The model under review builds one solid part; all positions refer to its coordinate system, in mm. A direction names the side the tool comes from. Give positions to 0.01 mm unless a question says otherwise; leave off trailing zeros. Write each loop counter-clockwise with the first axis right and the second up, starting at its lowest first coordinate (ties: lowest second). Pieces come first, ordered by that corner, then holes. Notation, with made-up numbers: (17.5, 11) - (44.5, 11) arc R24 ccw to (44.5, 41) - close; hole circle Ø9 at (82, -36). An arc over 180 degrees is marked (long way). Write item = value, one per line.
```python
from build123d import *

# Parameters (mm, degrees)
BOSS_EXTRUDE1_DEPTH = 1.8
FILLET1_R           = 0.5
SKETCH2_R           = 1.75
BOSS_EXTRUDE3_DEPTH = 1.8
FILLET2_R           = 3


with BuildPart() as part:
    # Sketch1 → Boss-Extrude1 (new body)
    with BuildSketch(Plane.XY):
        with BuildLine():
            Line((0, 4.5), (0, 6.5))
            Line((0, 6.5), (6, 6.5))
            Line((6, 6.5), (6, 10.5))
            Line((6, 10.5), (10, 14.5))
            Line((10, 14.5), (10, 83.5))
            Line((10, 83.5), (16.4, 83.5))
            ThreePointArc((16.4, 83.5), (17.2719581, 81.425344658), (17.601960582, 79.199226044))
            Line((17.601960582, 79.199226044), (18.25, 49.5))
            Line((18.25, 49.5), (12, 49.5))
            Line((12, 49.5), (12, 37))
            add(Edge.make_bspline(
                [(12, 37), (12, 35.742192932), (12.5, 34.153450807), (12.5, 32.15)],
                knots=[0, 0, 0, 0, 1, 1, 1, 1], degree=3))
            Line((12.5, 32.15), (12.5, 2.89))
            ThreePointArc((12.5, 2.89), (11.653538598, 0.846461402), (9.61, 0))
            ThreePointArc((9.61, 0), (4.304293167, 1.180712741), (0, 4.5))
        make_face()
    extrude(amount=BOSS_EXTRUDE1_DEPTH)

    # Fillet1
    fillet1_edges = [part.edges().sort_by_distance(p)[0] for p in [
        (0, 4.5, 0.9),
        (0, 6.5, 0.9),
        (6, 6.5, 0.9),
        (6, 10.5, 0.9),
        (10, 14.5, 0.9),
        (10, 83.5, 0.9),
        (18.25, 49.5, 0.9),
        (12, 49.5, 0.9),
    ]]
    fillet(fillet1_edges, radius=FILLET1_R)

    # Sketch2 → Boss-Extrude3 (add)
    with BuildSketch(Plane.XY):
        with BuildLine():
            Line((7, -2.499596966), (7, 0.500403034))
            Line((7, 0.500403034), (11, 0.500403034))
            Line((11, 0.500403034), (11.824045318, -1.578286292))
            ThreePointArc((11.824045318, -1.578286292), (9.968981185, -4.955214332), (7, -2.499596966))
        make_face()
        with Locations((9.5, -2.499596966)):
            Circle(SKETCH2_R, mode=Mode.SUBTRACT)
    extrude(amount=BOSS_EXTRUDE3_DEPTH)

    # Fillet2
    fillet2_edges = [part.edges().sort_by_distance(p)[0] for p in [
        (16.4, 83.5, 0.9),
    ]]
    fillet(fillet2_edges, radius=FILLET2_R)


solid = part.part
```
1. Insertion check: P1, Ø0.9, axis at x = 16.5, z = 1, coming from the -Y side; P2, Ø0.5, axis at y = 9, z = 1, coming from the -X side; P3, Ø0.5, axis at y = -1.5, z = 1, coming from the -X side. Each pin has a flat end and moves straight along its axis. Give the tip position at first contact, or say it passes through.
Findings below:
P1 = 49.5
P2 = 6
P3 = 7
2. Take a section at A-A on y = 38. Give the boundary of the cut face in (x, z), and give its area (3 significant figures).
Findings below:
outline = (10, 0) - (12, 0) - (12, 1.8) - (10, 1.8) - close
area = 3.60 mm²
3. For line 1 (Y direction, x = 9.25, z = 0.95); line 2 (X direction, y = 32.5, z = 0.6) (3 decimals); line 3 (Y direction, x = 9.5, z = 1.35), list the stretches that pass through material, from the lowest coordinate up. Write a range as from..to.
Findings below:
line_1 = -4.99..-4.23, -0.77..13.75
line_2 = 10..12.495
line_3 = -5..-4.25, -0.75..14
4. Take a section at B-B on x = 3. Give the boundary of the cut face in (y, z).
Findings below:
outline = (1.89, 0) - (6.5, 0) - (6.5, 1.8) - (1.89, 1.8) - close
5. Draft analysis for pull direction Y (two halves, no side actions). For faces 1 (the flat face through (11.43, -0.58, 0.89)), 2 (the flat face through (8, 12.5, 0.9)), 3 (the flat face through (7, -1, 1)), state which applies: +Y half, -Y half, draft (parallel to the pull), parting line (faces both ways), or undercut.
Findings below:
face_1 = undercut
face_2 = +Y half
face_3 = draft
6. Machinability: for faces 4 (the flat face through (12, 43, 1)), 5 (the flat face through (10, 48, 1)), 6 (the flat face through (15, 49.5, 1)), 7 (the cylindrical face through (17.518, 80.246, 0.887)), which of the approach directions +Z, -Z, +X, -X, +Y, -Y give a long, thin tool a straight path to every point of the face, cutting with its end or side? Answer none if there is none.
Findings below:
face_4 = +Z, -Z, +X
face_5 = +Z, -Z, -X, +Y
face_6 = +Z, -Z, +X, -Y
face_7 = +Z, -Z, +X, +Y
